Autodesk Inventor part; units mm, degrees
ref_plane "YZ Plane" through (0, 0, 0) normal (1, 0, 0) x (0, 1, 0)
ref_plane "XZ Plane" through (0, 0, 0) normal (0, 1, 0) x (-1, 0, 0)
ref_plane "XY Plane" through (0, 0, 0) normal (0, 0, 1) x (1, 0, 0)
sketch "Esboço1" plane through (0, 0, 0) normal (0, 0, 1) x (1, 0, 0)
  circle A0 centre (0, 0) radius 5
  dimension "d0" = 10
extrude "Extrusão1" add sketch "Esboço1" along normal blind 1
sketch "Esboço2" plane through (0, 0, 1) normal (0, 0, 1) x (1, 0, 0)
  circle A0 centre (0, 0) radius 4
  dimension "d3" = 8
extrude "Extrusão2" add sketch "Esboço2" along normal blind 1
sketch "Esboço3" plane through (0, 0, 2) normal (0, 0, 1) x (1, 0, 0)
  circle A0 centre (0, 0) radius 5
  dimension "d6" = 10
extrude "Extrusão3" add sketch "Esboço3" along normal blind 1
sketch "Esboço4" plane through (0, 0, 3) normal (0, 0, 1) x (1, 0, 0)
  circle A0 centre (0, 0) radius 4
  circle A1 centre (0, 0) radius 1
  dimension "d9" = 2
extrude "Extrusão4" cut sketch "Esboço4" against normal blind 4 contours A1
thread "Rosca1"
sketch "Esboço5" plane through (0, 0, 3) normal (0, 0, 1) x (1, 0, 0)
  circle A0 centre (0, 0) radius 5
  line L0 (-4, 0) -> (-4, -0.5)
  circle A1 centre (0, 0) radius 4
  line L1 (-4, 0) -> (-3.5, 0) construction
  line L2 (-4, -0.5) -> (-5, -0.5)
  line L3 (-5, -0.5) -> (-5, 0.5)
  line L4 (-5, -0.5) -> (-4, -0.5) construction
  line L5 (-5, 0.5) -> (-4, 0.5)
  line L6 (-4, 0.5) -> (-4, 0)
  line L7 (-4, -0.5) -> (-5, -0.5)
  dimension "d15" = 0.5
  dimension "d16" = 90
  dimension "d17" = 1
  dimension "d18" = 90
extrude "Extrusão5" cut sketch "Esboço5" against normal blind 10 contours L5 L6 L0 L2 A0 | A0 L3 L5 | L2 L3 A0 picked at (-4.3296, -0.2779)
sketch "Esboço7" plane through (0, 0, 3) normal (0, 0, 1) x (1, 0, 0)
  circle A0 centre (0, 0) radius 1
  circle A1 centre (0, 0) radius 1
  circle A2 centre (0, 0) radius 8.5
  line L0 (-8.5, 0) -> (-7.5, 0)
  line L1 (-7.5, 0) -> (-7.5, -0.5)
  line L2 (-7.5, -0.5) -> (-8.4853, -0.5)
  line L3 (-7.5, 0) -> (-7.5, 0.5)
  line L4 (-7.5, 0.5) -> (-8.4853, 0.5)
  dimension "d21" = 17
  dimension "d22" = 1
  dimension "d23" = 0.5
  dimension "d24" = 0.5
extrude "Extrusão6" add sketch "Esboço7" against normal blind 1 contours A2 L2 L1 L3 L4
sketch "Esboço8" plane through (0, 0, 2) normal (0, 0, -1) x (-1, 0, 0)
  circle A0 centre (0, 0) radius 1
  circle A1 centre (0, 0) radius 1
  circle A2 centre (0, 0) radius 7.5
  dimension "d27" = 15
extrude "Extrusão7" add sketch "Esboço8" along normal blind 1
sketch "Esboço9" plane through (0, 0, 0) normal (0, 0, -1) x (-1, 0, 0)
  circle A0 centre (0, 0) radius 1
  circle A1 centre (0, 0) radius 8.5
  line L0 (8.4853, -0.5) -> (7.5, -0.5)
  line L1 (7.5, 0) -> (7.5, -0.5)
  line L2 (7.5, -0.5) -> (8.4853, -0.5)
  line L3 (8.4853, -0.5) -> (8.4853, 0.5)
  line L4 (8.4853, 0.5) -> (7.5, 0.5)
  line L5 (7.5, 0.5) -> (8.4853, 0.5)
  line L6 (7.5, -0.5) -> (7.5, 0.5)
extrude "Extrusão8" add sketch "Esboço9" against normal blind 1 contours L4 L6 L1 L0 A1
properties part number "Polia2"
Can you work these out from the model? Positions are in its coordinate system, mm. A direction names the side the tool comes from. Coordinates: 2 decimals unless noted, no trailing zeros. Loops run counter-clockwise (first coordinate to the right, second up) from the corner with the lowest first, then second, coordinate; pieces in that order, holes last. Notation, with made-up numbers: M -1.75,-30.75 L 30.25,-30.75 A21 ccw 30.25,-13.75 Z; hole C 25.25,22.25 d5. An arc over 180 degrees is marked long. Put each result on its own line as item: value. Start each with the question number.
(1) Will these pins go through, and if not, where does the flat tip stop? pin 1 Ø1.5 at (x, z) = (4, 2) entering from -Y; pin 2 Ø0.5 at (x, z) = (-8, 2.5) entering from +Y; pin 3 Ø1.5 at (x, z) = (1.5, 1.5) entering from -Y.
(2) I need wall thicknesses on probe 1 along Z at (x, y) = (-5.75, 5); probe 2 along Y at (x, z) = (0, 1.4); probe 3 along X at (y, z) = (-6.5, 2.65). Which ranges of each line are inside material? Lowest first, please.
(3) Imagine slicing it at A-A on x = 0. List the corners of the cut face in (y, z) for me, and give its area (3 significant figures).
(4) Which directions (+Z, -Z, +X, -X, +Y, -Y) give clear straight access to the entire face, cutting with the end or side of a thin tool? Please do faces 5 (the face through (-8, -0.5, 2.5)), 6 (the face through (5, -6, 2)), 7 (the face through (0, -2, 3)).
(5) We'd pull the mould along Y, two halves only. Please class faces 1 (the face through (8.49, 0.37, 0.49)), 2 (the face through (-8, 0.5, 0.5)), 3 (the face through (-2, 0, 0)), 4 (the face through (-8, 0.5, 2.5)): +Y half, -Y half, draft (parallel to the pull), parting line (faces both ways), or undercut.
(6) Imagine slicing it at D-D on x = 4.75. List the corners of the cut face in (y, z) for me.
(7) Imagine slicing it at B-B on y = 7.75. List the corners of the cut face in (x, z) for me, and give its area (3 significant figures).
(8) Imagine slicing it at C-C on z = 0.35. List the corners of the cut face in (x, y) for me.
Worked answers:
1. pin 1: stops at y = -7.85
1. pin 2: stops at y = 3.49
1. pin 3: stops at y = -8.45
2. probe 1: z = 0 to 1, 2 to 3
2. probe 2: y = -7.5 to -1, 1 to 7.5
2. probe 3: x = -5.48 to 5.48
3. outline: M -8.5,0 L -1,0 L -1,3 L -8.5,3 L -8.5,2 L -7.5,2 L -7.5,1 L -8.5,1 Z; M 1,0 L 8.5,0 L 8.5,1 L 7.5,1 L 7.5,2 L 8.5,2 L 8.5,3 L 1,3 Z
3. area: 43.0 mm2
4. face 5: +Z, -Z, -X
4. face 6: none
4. face 7: +Z, +X, -X, +Y, -Y
5. face 1: parting line
5. face 2: undercut
5. face 3: draft
5. face 4: undercut
6. outline: M -7.05,0 L 7.05,0 L 7.05,1 L 5.8,1 L 5.8,2 L 7.05,2 L 7.05,3 L -7.05,3 L -7.05,2 L -5.8,2 L -5.8,1 L -7.05,1 Z
7. outline: M -3.49,0 L 3.49,0 L 3.49,1 L -3.49,1 Z; M -3.49,2 L 3.49,2 L 3.49,3 L -3.49,3 Z
7. area: 14.0 mm2
8. outline: M -8.49,-0.5 A8.5 ccw long -8.49,0.5 L -7.5,0.5 L -7.5,-0.5 Z; hole C 0,0 d2
